Design review of the part built by this model. Coordinates are the model's own, in mm. Give positions to 0.01 mm unless a question says otherwise; leave off trailing zeros. Write each loop counter-clockwise with the first axis right and the second up, starting at its lowest first coordinate (ties: lowest second). Pieces come first, ordered by that corner, then holes. Notation, with made-up numbers: (-6, -39) -> (50, -39) arc R18 cw to (50, -27) -> close; hole circle Ø9 at (87.5, 82.5). An arc over 180 degrees is marked (long way). Write each question's results on one line, items separated by ' | '. Start each with the question number.
(1) To check wall thickness, follow probe 1 along X at (y, z) = (83, 8); probe 2 along Y at (x, z) = (115, 5.5); probe 3 along X at (y, z) = (-1, 4.25). State the ranges of each line that lie inside material, in increasing order.
(2) Take a section at A-A (y = 78). State the section outline as (x, z) points.
(3) Take a section at C-C (x = 60.5). State the section outline as (y, z) points.
(4) Take a section at B-B (z = 5). State the section outline as (x, y) points, plus the area to 3 significant figures.
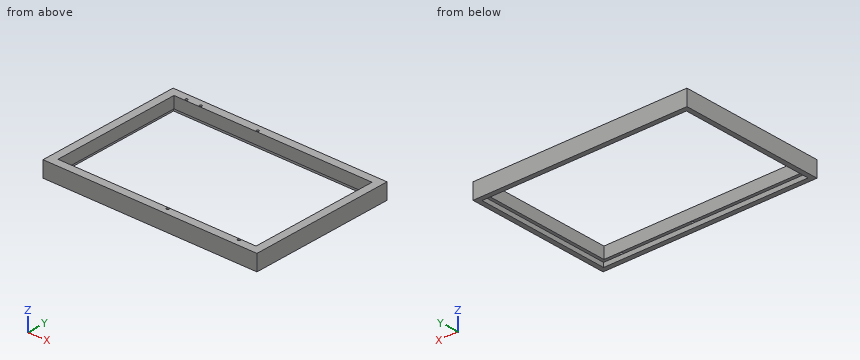
from build123d import *

# Parameters (mm, degrees)
SKETCH_1_W           = 135
SKETCH_1_H           = 92
SKETCH_1_R           = 0.8
SKETCH_1_W_2         = 125
SKETCH_1_H_2         = 82
EXTRUDE_1_DEPTH      = 10
EXTRUDE_1_DEPTH_BACK = 0.0001
SKETCH_4_W           = 129
SKETCH_4_H           = 86
CUT_EXTRUDE_1_DEPTH  = 2.75


with BuildPart() as part:
    # Эскиз1 → Бобышка-Вытянуть1 (new body, two sides)
    with BuildSketch(Plane.XY) as extrude_1_sk:
        with Locations((62.5, 41)):
            Rectangle(SKETCH_1_W, SKETCH_1_H)
        with Locations((7, 83)):
            Circle(SKETCH_1_R, mode=Mode.SUBTRACT)
        with Locations((115, -1)):
            Circle(SKETCH_1_R, mode=Mode.SUBTRACT)
        with Locations((16, 83)):
            Circle(SKETCH_1_R, mode=Mode.SUBTRACT)
        with Locations((52, 83)):
            Circle(SKETCH_1_R, mode=Mode.SUBTRACT)
        with Locations((70.05, -1)):
            Circle(SKETCH_1_R, mode=Mode.SUBTRACT)
        with Locations((62.5, 41)):
            Rectangle(SKETCH_1_W_2, SKETCH_1_H_2, mode=Mode.SUBTRACT)
    extrude(amount=EXTRUDE_1_DEPTH)
    extrude(extrude_1_sk.sketch, amount=-EXTRUDE_1_DEPTH_BACK)

    # Эскиз4 → Вырез-Вытянуть1 (cut)
    with BuildSketch(Plane(origin=(0, 0, -0.0001), x_dir=(-1, 0, 0), z_dir=(0, 0, -1))):
        with Locations((-62.5, 41)):
            Rectangle(SKETCH_4_W, SKETCH_4_H)
    extrude(amount=-CUT_EXTRUDE_1_DEPTH, mode=Mode.SUBTRACT)


solid = part.part
Report:
1) probe 1: -5 to 6.2, 7.8 to 15.2, 16.8 to 51.2, 52.8 to 130 | probe 2: -5 to -1.8, -0.2 to 0, 82 to 87 | probe 3: -5 to 69.25, 70.85 to 114.2, 115.8 to 130
2) outline: (-5, 0) -> (-2, 0) -> (-2, 2.75) -> (0, 2.75) -> (0, 10) -> (-5, 10) -> close; (125, 2.75) -> (127, 2.75) -> (127, 0) -> (130, 0) -> (130, 10) -> (125, 10) -> close
3) outline: (-5, 0) -> (-2, 0) -> (-2, 2.75) -> (0, 2.75) -> (0, 10) -> (-5, 10) -> close; (82, 2.75) -> (84, 2.75) -> (84, 0) -> (87, 0) -> (87, 10) -> (82, 10) -> close
4) outline: (-5, -5) -> (130, -5) -> (130, 87) -> (-5, 87) -> close; hole (0, 0) -> (125, 0) -> (125, 82) -> (0, 82) -> close; hole circle Ø1.6 at (7, 83); hole circle Ø1.6 at (16, 83); hole circle Ø1.6 at (52, 83); hole circle Ø1.6 at (70.05, -1); hole circle Ø1.6 at (115, -1) | area: 2,160 mm2
